Source: CAD feature listing. Evaluate the final solid. Frame: model axes, mm. A direction names the side the tool comes from. Give positions to 0.01 mm unless a question says otherwise; leave off trailing zeros. Write each loop counter-clockwise with the first axis right and the second up, starting at its lowest first coordinate (ties: lowest second). Pieces come first, ordered by that corner, then holes. Notation, with made-up numbers: (-26.5, -14) -> (-13.5, -14) arc R18 ccw to (-13.5, -9) -> close; hole circle Ø1 at (-11.75, -21). An arc over 180 degrees is marked (long way). Use a Markdown table: item, result. Add a question column.
```python
from build123d import *
from OCP.BRepFilletAPI import BRepFilletAPI_MakeChamfer

# Parameters (mm, degrees)
RESSALTO_EXTRUS_O1_DEPTH = 3
RESSALTO_EXTRUS_O2_DEPTH = 32
FILETE1_R                = 1
CHANFRO1_SIZE            = 0.5
CHANFRO1_SIZE_2          = 0.499987399
CHANFRO1_SIZE_3          = 0.499991089
FILETE10_R               = 0.4


with BuildPart() as part:
    # Esboço1 → Ressalto-extrusão1 (new body)
    with BuildSketch(Plane.XY):
        Polygon((5.893734702, -9.900463955), (6.106086441, 19.167541422), (34.606086441, 19.167541422), (34.606086441, -15.232458579), (-35.393913559, -15.232458579), (-35.393913559, -9.89942335), align=None)
        Polygon((10.891442786, -10.232458579), (11.069693146, 14.167541422), (29.606086441, 14.167541422), (29.606086441, -10.232458579), align=None, mode=Mode.SUBTRACT)
        with BuildLine():
            Line((-31.393913559, -11.201458579), (-26.393913559, -11.201458579))
            ThreePointArc((-26.393913559, -11.201458579), (-24.893913559, -12.701458579), (-26.393913559, -14.201458579))
            Line((-26.393913559, -14.201458579), (-31.393913559, -14.201458579))
            ThreePointArc((-31.393913559, -14.201458579), (-32.893913559, -12.701458579), (-31.393913559, -11.201458579))
        make_face(mode=Mode.SUBTRACT)
        with BuildLine():
            Line((-15.393913559, -11.201458579), (-10.393913559, -11.201458579))
            ThreePointArc((-10.393913559, -11.201458579), (-8.893913559, -12.701458579), (-10.393913559, -14.201458579))
            Line((-10.393913559, -14.201458579), (-15.393913559, -14.201458579))
            ThreePointArc((-15.393913559, -14.201458579), (-16.893913559, -12.701458579), (-15.393913559, -11.201458579))
        make_face(mode=Mode.SUBTRACT)
    extrude(amount=RESSALTO_EXTRUS_O1_DEPTH)

    # Esboço2 → Ressalto-extrusão2 (add)
    with BuildSketch(Plane.ZY.offset(35.393913559)):
        Polygon((0, -15.232458579), (-2.486055277, -17.718513856), (0.513944723, -17.718513856), (3, -15.232458579), align=None)
    extrude(amount=-RESSALTO_EXTRUS_O2_DEPTH)

    # Filete1
    filete1_edges = [part.edges().sort_by_distance(p)[0] for p in [
        (5.999910572, 4.633538733, 0),
        (20.356086441, 19.167541422, 0),
        (34.606086441, 1.967541422, 0),
        (-14.750089428, -9.899943653, 0),
        (29.606086441, 1.967541422, 0),
        (20.337889794, 14.167541422, 0),
        (10.980567966, 1.967541422, 0),
        (20.248764614, -10.232458579, 0),
        (6.106086441, 19.167541422, 1.5),
        (34.606086441, 19.167541422, 1.5),
        (34.606086441, -15.232458579, 1.5),
        (29.606086441, -10.232458579, 1.5),
        (29.606086441, 14.167541422, 1.5),
        (11.069693146, 14.167541422, 1.5),
        (10.891442786, -10.232458579, 1.5),
        (20.248764614, -10.232458579, 3),
        (10.980567966, 1.967541422, 3),
        (15.606086441, -15.232458579, 0),
        (15.606086441, -15.232458579, 3),
        (20.337889794, 14.167541422, 3),
        (29.606086441, 1.967541422, 3),
        (-14.750089428, -9.899943653, 3),
        (34.606086441, 1.967541422, 3),
        (20.356086441, 19.167541422, 3),
        (5.999910572, 4.633538733, 3),
    ]]
    fillet(filete1_edges, radius=FILETE1_R)

    # Chanfro1
    chanfro1_edges_1 = [part.edges().sort_by_distance(p)[0] for p in [
        (-35.393913559, -9.89942335, 1.5),
    ]]
    chanfro1_side_1 = [part.faces().sort_by_distance(p)[0] for p in [
        (-35.383913811, -9.899423602, 1.5),
    ]]
    chanfro1_edges_2 = [part.edges().sort_by_distance(p)[0] for p in [
        (-35.393895737, -10.19231657, 0.292893219),
    ]]
    chanfro1_side_2 = [part.faces().sort_by_distance(p)[0] for p in [
        (-35.393895737, -10.199387512, 0.299964161),
    ]]
    chanfro1_edges_3 = [part.edges().sort_by_distance(p)[0] for p in [
        (-35.393895737, -10.19231657, 2.707106781),
    ]]
    chanfro1_side_3 = [part.faces().sort_by_distance(p)[0] for p in [
        (-35.393895737, -10.199387512, 2.700035839),
    ]]
    chanfro1_edges_4 = [part.edges().sort_by_distance(p)[0] for p in [
        (-35.393913559, -13.065940965, 0),
        (-35.393913559, -13.065940965, 3),
    ]]
    chanfro1 = BRepFilletAPI_MakeChamfer(part.part.solid().wrapped)
    for e in chanfro1_edges_1:
        chanfro1.Add(CHANFRO1_SIZE, CHANFRO1_SIZE_2, e.wrapped, chanfro1_side_1[0].wrapped)
    for e in chanfro1_edges_2:
        chanfro1.Add(CHANFRO1_SIZE, CHANFRO1_SIZE_3, e.wrapped, chanfro1_side_2[0].wrapped)
    for e in chanfro1_edges_3:
        chanfro1.Add(CHANFRO1_SIZE, CHANFRO1_SIZE_3, e.wrapped, chanfro1_side_3[0].wrapped)
    for e in chanfro1_edges_4:
        chanfro1.Add(CHANFRO1_SIZE, e.wrapped)
    add(Compound.cast(chanfro1.Shape()), mode=Mode.REPLACE)
    chanfro1_2_edges = [part.edges().sort_by_distance(p)[0] for p in [
        (-35.393913559, -16.475486217, -1.243027639),
    ]]
    chamfer(chanfro1_2_edges, length=CHANFRO1_SIZE)
    chanfro1_3_edges = [part.edges().sort_by_distance(p)[0] for p in [
        (-35.393913559, -16.725479917, 1.506978662),
    ]]
    chamfer(chanfro1_3_edges, length=CHANFRO1_SIZE)
    chanfro1_4_edges = [part.edges().sort_by_distance(p)[0] for p in [
        (-35.393913559, -17.718513856, -0.986055277),
    ]]
    chamfer(chanfro1_4_edges, length=CHANFRO1_SIZE)
    chanfro1_5_edges = [part.edges().sort_by_distance(p)[0] for p in [
        (-3.393913559, -14.732458579, 3),
    ]]
    chamfer(chanfro1_5_edges, length=CHANFRO1_SIZE)
    chanfro1_6_edges = [part.edges().sort_by_distance(p)[0] for p in [
        (-3.393913559, -16.475486217, -1.243027639),
    ]]
    chamfer(chanfro1_6_edges, length=CHANFRO1_SIZE)
    chanfro1_7_edges = [part.edges().sort_by_distance(p)[0] for p in [
        (-3.393913559, -16.725486217, 1.506972361),
    ]]
    chamfer(chanfro1_7_edges, length=CHANFRO1_SIZE)
    chanfro1_8_edges = [part.edges().sort_by_distance(p)[0] for p in [
        (-3.393913559, -17.718513856, -0.986055277),
    ]]
    chamfer(chanfro1_8_edges, length=CHANFRO1_SIZE)
    chanfro1_9_edges = [part.edges().sort_by_distance(p)[0] for p in [
        (-3.393913559, -14.732458579, 0),
    ]]
    chamfer(chanfro1_9_edges, length=CHANFRO1_SIZE)

    # Filete10
    filete10_edges = [part.edges().sort_by_distance(p)[0] for p in [
        (-19.393913559, -17.718513856, -2.486055277),
    ]]
    fillet(filete10_edges, radius=FILETE10_R)


solid = part.part
```
(1) First-contact query: pin 1 Ø1.1 at (y, z) = (-16, -0.5) entering from +X; pin 2 Ø1.5 at (x, z) = (-12.5, 2) entering from +Y; pin 3 Ø0.9 at (x, z) = (-29, 1) entering from -Y. Flat tips, straight axial feed; report the tip coordinate or a pass-through.
(2) Material intervals for L1, parallel to X at y = -12.5, z = 2.1; L2, parallel to Y at x = 25, z = 1.75; L3, parallel to Y at x = 31, z = 1.6, sorted ascending.
(3) Mould query, pull axis X, two halves, no side actions, for faces 6 (the cylindrical face through (-8.894, -12.668, 1.479)), 7 (the flat face through (-35.14, -16.38, -0.8)), 8 (the flat face through (-3.64, -16.355, -0.764)), 9 (the cylindrical face through (-32.894, -12.734, 1.479)). Classes: +X half, -X half, draft (parallel to the pull), parting line (faces both ways), or undercut.
(4) Cut plane A-A on x = 24. Return the cut outline in (y, z), then the cut area to 3 significant figures.
(5) Access query for faces 1 (the flat face through (-29, -14.201, 1)), 2 (the flat face through (9.7, -2.2, 0)), 3 (the cylindrical face through (6.29, 3.84, 0.29)), 4 (the cylindrical face through (6.28, 3.84, 2.7)), 5 (the flat face through (-19.61, -16.49, 1.74)). Directions: +Z, -Z, +X, -X, +Y, -Y. A direction counts if a zero-diameter tool reaches every point of the face in a straight line with its end or side. Return the directions, or none.
(6) Cut plane C-C on x = 8. Return the cut outline in (y, z), then the cut area to 3 significant figures.
(7) Cut plane B-B on y = -12. Return the cut outline in (x, z).
Output:
| question | item | result |
|---|---|---|
| 1 | pin 1 | x = -3.39 |
| 1 | pin 2 | y = -9.9 |
| 1 | pin 3 | y = -17.68 |
| 2 | L1 | -35.39 to -32.88, -24.91 to -16.88, -8.91 to 34.6 |
| 2 | L2 | -15.23 to -10.23, 14.17 to 19.17 |
| 2 | L3 | -15.23 to 19.17 |
| 3 | face 6 | undercut |
| 3 | face 7 | -X half |
| 3 | face 8 | +X half |
| 3 | face 9 | undercut |
| 4 | outline | (-15.23, 1) arc R1 ccw to (-14.23, 0) -> (-11.23, 0) arc R1 ccw to (-10.23, 1) -> (-10.23, 2) arc R1 ccw to (-11.23, 3) -> (-14.23, 3) arc R1 ccw to (-15.23, 2) -> close; (14.17, 1) arc R1 ccw to (15.17, 0) -> (18.17, 0) arc R1 ccw to (19.17, 1) -> (19.17, 2) arc R1 ccw to (18.17, 3) -> (15.17, 3) arc R1 ccw to (14.17, 2) -> close |
| 4 | area | 28.3 mm^2 |
| 5 | face 1 | +Z, -Z |
| 5 | face 2 | -Z, +X, -X, +Y |
| 5 | face 3 | -Z, -X, +Y |
| 5 | face 4 | +Z, -X, +Y |
| 5 | face 5 | +Z, +X, -X, -Y |
| 6 | outline | (-15.23, 1) arc R1 ccw to (-14.23, 0) -> (18.17, 0) arc R1 ccw to (19.17, 1) -> (19.17, 2) arc R1 ccw to (18.17, 3) -> (-14.23, 3) arc R1 ccw to (-15.23, 2) -> close |
| 6 | area | 102 mm^2 |
| 7 | outline | (-35.39, 0.5) -> (-34.89, 0) -> (-32.72, 0) -> (-32.72, 3) -> (-34.89, 3) -> (-35.39, 2.5) -> close; (-25.07, 0) -> (-16.72, 0) -> (-16.72, 3) -> (-25.07, 3) -> close; (-9.07, 0) -> (33.61, 0) arc R1 ccw to (34.61, 1) -> (34.61, 2) arc R1 ccw to (33.61, 3) -> (-9.07, 3) -> close |
